Could you check a few things on this model? Use its own coordinates, in mm. Give positions to 0.01 mm unless a question says otherwise; leave off trailing zeros. Order: outer loops, then holes, each group sorted by start corner. A loop starts at its lowest first (then second) coordinate and runs counter-clockwise, first axis right, second up. Notation, with made-up numbers: M 7.25,12.25 L 37.25,12.25 A12 ccw 37.25,22.25 Z; hole C -28.75,45 d5. An arc over 180 degrees is marked long. Return JSON: item names as keys, results as strings. Group by question number.
```python
from build123d import *

# Parameters (mm, degrees)
ESQUISSE1_W        = 10
ESQUISSE1_H        = 10
BOSS_EXTRU_1_DEPTH = 6
CHANFREIN1_SIZE    = 3
CHANFREIN2_SIZE    = 1


with BuildPart() as part:
    # Esquisse1 → Boss.-Extru.1 (new body)
    with BuildSketch(Plane(origin=(0, 0, 0), x_dir=(1, 0, 0), z_dir=(0, 1, 0))):
        Rectangle(ESQUISSE1_W, ESQUISSE1_H)
    extrude(amount=BOSS_EXTRU_1_DEPTH)

    # Chanfrein1
    chanfrein1_edges = [part.edges().sort_by_distance(p)[0] for p in [
        (0, 0, 5),
        (-5, 0, 0),
        (0, 0, -5),
        (5, 0, 0),
    ]]
    chamfer(chanfrein1_edges, length=CHANFREIN1_SIZE)

    # Chanfrein2
    chanfrein2_edges = [part.edges().sort_by_distance(p)[0] for p in [
        (5, 4.5, 5),
        (-5, 4.5, 5),
        (-5, 4.5, -5),
        (5, 4.5, -5),
    ]]
    chamfer(chanfrein2_edges, length=CHANFREIN2_SIZE)


solid = part.part
```
1. Imagine slicing it at B-B, the plane y = 5.6. Please give me the cut outline in (x, z), plus the area to 3 significant figures.
2. Imagine slicing it at C-C, the plane z = 1.5. Please give me the cut outline in (x, y).
3. Imagine slicing it at D-D, the plane y = 2.8. Please give me the cut outline in (x, z), plus the area to 3 significant figures.
4. For pin 1 (2 mm diameter, centred on x = 3.5, z = -1.5, fed in from -Y); pin 2 (2 mm diameter, centred on x = -1, y = 2.5, fed in from -Z), each with a flat end and sliding along its axis, tell me the tip position at first contact or that it passes through.
5. Imagine slicing it at A-A, the plane x = 3.75. Please give me the cut outline in (y, z), plus the area to 3 significant figures.
6. I need wall thicknesses on L1, parallel to Y at x = -3, z = 4.5; L2, parallel to Z at x = 4.5, y = 3.7; L3, parallel to Y at x = -4, z = 3.25. Which ranges of each line are inside material? Lowest first, please. Write a range as from..to.
Values:
{
 "1": {"outline": "M -5,-4 L -4,-5 L 4,-5 L 5,-4 L 5,4 L 4,5 L -4,5 L -5,4 Z", "area": "98.0 mm²"},
 "2": {"outline": "M -5,3 L -2,0 L 2,0 L 5,3 L 5,6 L -5,6 Z"},
 "3": {"outline": "M -4.8,-4.2 L -4.2,-4.8 L 4.2,-4.8 L 4.8,-4.2 L 4.8,4.2 L 4.2,4.8 L -4.2,4.8 L -4.8,4.2 Z", "area": "91.4 mm²"},
 "4": {"pin 1": "stops at y = 0.5", "pin 2": "stops at z = -5"},
 "5": {"outline": "M 1.75,-3.75 L 3,-5 L 6,-5 L 6,5 L 3,5 L 1.75,3.75 Z", "area": "40.9 mm²"},
 "6": {"L1": "y = 2.5..6", "L2": "z = -4.5..4.5", "L3": "y = 2..6"}
}
